```python
from build123d import *

# Parameters (mm, degrees)
LOFT_THIN1_OUTLINE_W      = 64
LOFT_THIN1_OUTLINE_H      = 36
LOFT_THIN1_OUTLINE_W_2    = 61
LOFT_THIN1_OUTLINE_H_2    = 33
LOFT_THIN1_DEPTH          = 5
SKETCH3_4_W               = 64
SKETCH3_4_H               = 36
SKETCH3_4_W_2             = 61
SKETCH3_4_H_2             = 33
EXTRUDE_THIN1_DEPTH       = 10
SKETCH8_W                 = 1.5
SKETCH8_H                 = 10
BOSS_EXTRUDE3_DEPTH       = 6
SKETCH7_W                 = 1.5
SKETCH7_H                 = 36
BOSS_EXTRUDE2_DEPTH       = 30
F_3_0MM_DOWEL_HOLE1_D     = 3.5
F_3_0MM_DOWEL_HOLE1_DEPTH = 7
F_3_0MM_DOWEL_HOLE1_TIP   = 1.051506083
FILLET1_R                 = 2
FILLET2_START             = -25
FILLET2_DEPTH             = 44


with BuildPart() as part:
    # Loft-Thin1: read off the stored shape, not the designer's step
    # Loft-Thin1 outline → Loft-Thin1 (new body)
    with BuildSketch(Plane.XY):
        Rectangle(LOFT_THIN1_OUTLINE_W, LOFT_THIN1_OUTLINE_H)
        Rectangle(LOFT_THIN1_OUTLINE_W_2, LOFT_THIN1_OUTLINE_H_2, mode=Mode.SUBTRACT)
    extrude(amount=LOFT_THIN1_DEPTH)

    # Sketch3<4> → Extrude-Thin1 (add)
    with BuildSketch(Plane.XY.offset(5)):
        Rectangle(SKETCH3_4_W, SKETCH3_4_H)
        Rectangle(SKETCH3_4_W_2, SKETCH3_4_H_2, mode=Mode.SUBTRACT)
    extrude(amount=EXTRUDE_THIN1_DEPTH)

    # Sketch8 → Boss-Extrude3 (add)
    with BuildSketch(Plane.XZ.offset(18)):
        with Locations((-31.25, 5)):
            Rectangle(SKETCH8_W, SKETCH8_H)
    extrude(amount=BOSS_EXTRUDE3_DEPTH)

    # Sketch7 → Boss-Extrude2 (add)
    with BuildSketch(Plane(origin=(32, 0, 0), x_dir=(0, 0, -1), z_dir=(1, 0, 0))):
        with Locations((-0.75, 0)):
            Rectangle(SKETCH7_W, SKETCH7_H)
    extrude(amount=BOSS_EXTRUDE2_DEPTH)

    # Ø3.0mm Dowel Hole1
    with Locations(Plane.ZY.offset(32)):
        with Locations((4, 1.8), (4, -18.5)):
            Hole(F_3_0MM_DOWEL_HOLE1_D / 2, depth=F_3_0MM_DOWEL_HOLE1_DEPTH)
            with Locations((0, 0, -(F_3_0MM_DOWEL_HOLE1_DEPTH + F_3_0MM_DOWEL_HOLE1_TIP / 2))):  # 118° drill point
                Cone(0, F_3_0MM_DOWEL_HOLE1_D / 2, F_3_0MM_DOWEL_HOLE1_TIP, mode=Mode.SUBTRACT)

    # Fillet1
    fillet1_edges = [part.edges().sort_by_distance(p)[0] for p in [
        (32, 0, 1.5),
    ]]
    fillet(fillet1_edges, radius=FILLET1_R)

    # Fillet2: read off the stored shape, not the designer's step
    # Fillet2 outline → Fillet2 (cut)
    with BuildSketch(Plane(origin=(0, 0, 0), x_dir=(1, 0, 0), z_dir=(0, 1, 0)).offset(FILLET2_START)):
        with BuildLine():
            Line((-32, 0), (-32, -1.5))
            ThreePointArc((-32, -1.5), (-31.560660172, -0.439339828), (-30.5, 0))
            Line((-30.5, 0), (-32, 0))
        make_face()
    extrude(amount=FILLET2_DEPTH, mode=Mode.SUBTRACT)


solid = part.part
```
Work out the finished part from the listing and answer in its coordinate system (mm). A direction names the side the tool comes from. Give positions to 0.01 mm unless a question says otherwise; leave off trailing zeros. Loops run counter-clockwise (first coordinate to the right, second up) from the corner with the lowest first, then second, coordinate; pieces in that order, holes last. Notation, with made-up numbers: (23, 3) -> (64, 3) arc R15 ccw to (64, 15) -> close; hole circle Ø2 at (-16, -26.5). An arc over 180 degrees is marked (long way). Put each result on its own line as item: value. Start each with the question number.
Item 1: Which of the six approach directions +Z, -Z, +X, -X, +Y, -Y give full straight-line access (tool end or side, diameter ignored) to faces 4 (the face through (48, 0, 1.5)), 5 (the face through (-30.5, 0, 7)), 6 (the face through (-29.229, -16.765, 4.228)), 7 (the face through (-30.5, -21, 5))?
Item 2: Find the intervals of material crossed by L1, parallel to Y at x = -31.15, z = 4; L2, parallel to X at y = 11.5, z = 10.5; L3, parallel to Y at x = 19, z = 14.5, in increasing order. Write a range as [from, to].
Item 3: Each of these flat-tipped pins is pushed along its axis until it touches: P1, Ø1.2, axis at x = -31.5, y = -19.5, coming from the +Z side; P2, Ø5, axis at y = -22.5, z = 7, coming from the +X side; P3, Ø9, axis at y = -2.5, z = 10.5, coming from the +X side. Where does it stop, or does it pass through?
Item 4: The part is cut by section C-C (x = 40). Give the vertices of the cut face in (y, z), then the cut area to 3 significant figures.
Item 5: The mould has two halves that part along Y. Classify faces 1 (the face through (32, 0, 9)), 2 (the face through (0, 16.5, 7)), 3 (the face through (4, 18, 8)): released by +Y, released by -Y, zero draft, split by the parting line, or undercut.
Item 6: The part is cut by section B-B (x = 17). Give the vertices of the cut face in (y, z).
Item 7: The part is cut by section A-A (y = 11). Give the vertices of the cut face in (x, z), then the cut area to 3 significant figures.
Answers below:
1. face 4: +Z, +X, +Y, -Y
1. face 5: +Z, -Z
1. face 6: -X
1. face 7: +Z, -Z, +X, -Y
2. L1: [-24, -20.25], [-16.75, 0.05], [3.55, 18]
2. L2: [-32, -30.5], [30.5, 32]
2. L3: [-18, -16.5], [16.5, 18]
3. P1: z = 10
3. P2: x = -30.5
3. P3: x = 32
4. outline: (-18, 0) -> (18, 0) -> (18, 1.5) -> (-18, 1.5) -> close
4. area: 54.0 mm2
5. face 1: zero draft
5. face 2: undercut
5. face 3: released by +Y
6. outline: (-18, 0) -> (-16.5, 0) -> (-16.5, 15) -> (-18, 15) -> close; (16.5, 0) -> (18, 0) -> (18, 15) -> (16.5, 15) -> close
7. outline: (-32, 1.5) arc R1.5 ccw to (-30.5, 0) -> (-30.5, 15) -> (-32, 15) -> close; (30.5, 0) -> (62, 0) -> (62, 1.5) -> (34, 1.5) arc R2 cw to (32, 3.5) -> (32, 15) -> (30.5, 15) -> close
7. area: 90.4 mm2
